from build123d import *

# Parameters (mm, degrees)
SKETCH1_W           = 60
SKETCH1_H           = 70
BOSS_EXTRUDE1_DEPTH = 5
SKETCH2_W           = 5
SKETCH2_H           = 70
BOSS_EXTRUDE2_DEPTH = 70
SKETCH3_R           = 2.5
CUT_EXTRUDE1_DEPTH  = 70
SKETCH4_R           = 11.5
CUT_EXTRUDE2_DEPTH  = 10
SKETCH5_R           = 1.5
CUT_EXTRUDE3_DEPTH  = 10


with BuildPart() as part:
    # Sketch1 → Boss-Extrude1 (new body)
    with BuildSketch(Plane(origin=(0, 0, 0), x_dir=(1, 0, 0), z_dir=(0, 1, 0))):
        Rectangle(SKETCH1_W, SKETCH1_H)
    extrude(amount=BOSS_EXTRUDE1_DEPTH)

    # Sketch2 → Boss-Extrude2 (add)
    with BuildSketch(Plane(origin=(0, 5, 0), x_dir=(1, 0, 0), z_dir=(0, 1, 0))):
        with Locations((27.5, 0)):
            Rectangle(SKETCH2_W, SKETCH2_H)
    extrude(amount=BOSS_EXTRUDE2_DEPTH)

    # Sketch3 → Cut-Extrude1 (cut)
    with BuildSketch(Plane(origin=(0, 5, 0), x_dir=(1, 0, 0), z_dir=(0, 1, 0))):
        with Locations(Location((0, 18.161512971, 0), (0, 0, 270))):
            Circle(SKETCH3_R)
        with Locations(Location((0, -18.161512971, 0), (0, 0, 90))):
            Circle(SKETCH3_R)
    extrude(amount=-CUT_EXTRUDE1_DEPTH, mode=Mode.SUBTRACT)

    # Sketch4 → Cut-Extrude2 (cut)
    with BuildSketch(Plane.ZY.offset(-25)):
        with Locations((0, 40)):
            Circle(SKETCH4_R)
    extrude(amount=-CUT_EXTRUDE2_DEPTH, mode=Mode.SUBTRACT)

    # Sketch5 → Cut-Extrude3 (cut)
    with BuildSketch(Plane.ZY.offset(-25)):
        with Locations((-15.5, 55.5)):
            Circle(SKETCH5_R)
        with Locations((15.5, 55.5)):
            Circle(SKETCH5_R)
        with Locations((15.5, 24.5)):
            Circle(SKETCH5_R)
        with Locations((-15.5, 24.5)):
            Circle(SKETCH5_R)
    extrude(amount=-CUT_EXTRUDE3_DEPTH, mode=Mode.SUBTRACT)


solid = part.part
Build history of the part. All positions in model axes, mm. A direction names the side the tool comes from. Coordinates: 2 decimals unless noted, no trailing zeros. Order: outer loops, then holes, each group sorted by start corner. A loop starts at its lowest first (then second) coordinate and runs counter-clockwise, first axis right, second up. Notation, with made-up numbers: M 78.5,1 L 97.5,1 A30 cw 97.5,40 Z; hole C 77,64.5 d6. An arc over 180 degrees is marked long. One line per question, with ' | ' between items. Start each with the question number.
Q1. Saw through at A-A (y = 55.5). List the corners of the cut face in (x, z).
Q2. Saw through at C-C (z = 0). List the corners of the cut face in (x, y), then the cut area to 3 significant figures.
Q3. 3-axis set-ups, long thin cutter, end or side, ignore diameter. For faces 1 (the face through (27.46, 55.57, -17)), 2 (the face through (25, 31.7, 8.3)): which of +Z, -Z, +X, -X, +Y, -Y reach the whole face in a straight line?
Q4. Probe L1, parallel to Y at x = 28.2, z = -15.5; L2, parallel to Y at x = 26.4, z = 0; L3, parallel to Y at x = 12.5, z = -4.5. List the from-to ranges inside material, lowest first. Write a range as from..to.
Q5. Saw through at B-B (y = 40). List the corners of the cut face in (x, z), then the cut area to 3 significant figures.
Q6. Saw through at D-D (z = -29). List the corners of the cut face in (x, y).
Q7. Two-plate mould, pull along X, no slides. Class faces 3 (the face through (-1.521, 2.535, -20.145)), 4 (the face through (1.521, 2.535, 20.145)), 5 (the face through (-30, 2, 0)), 6 (the face through (27, 21, 35)): +X half, -X half, draft (parallel to the pull), parting line (faces both ways), or undercut.
Q8. Flat gauge pins, fed straight in: pin 1 Ø3 at (x, z) = (23, 8) entering from -Y; pin 2 Ø20.5 at (y, z) = (40, 0) entering from +X; pin 3 Ø12 at (x, z) = (9.5, 1.5) entering from +Y; pin 4 Ø5 at (y, z) = (55.5, -15.5) entering from -X. Where does each tip first touch, or does it go through?
Check values:
1) outline: M 25,-35 L 30,-35 L 30,-17 L 25,-17 Z; M 25,-14 L 30,-14 L 30,14 L 25,14 Z; M 25,17 L 30,17 L 30,35 L 25,35 Z
2) outline: M -30,0 L 30,0 L 30,28.5 L 25,28.5 L 25,5 L -30,5 Z; M 25,51.5 L 30,51.5 L 30,75 L 25,75 Z | area: 535 mm2
3) face 1: +X, -X | face 2: +Z, -Z, -X, +Y
4) L1: y = 0..23, 26..54, 57..75 | L2: y = 0..28.5, 51.5..75 | L3: y = 0..5
5) outline: M 25,-35 L 30,-35 L 30,-11.5 L 25,-11.5 Z; M 25,11.5 L 30,11.5 L 30,35 L 25,35 Z | area: 235 mm2
6) outline: M -30,0 L 30,0 L 30,75 L 25,75 L 25,5 L -30,5 Z
7) face 3: undercut | face 4: undercut | face 5: -X half | face 6: draft
8) pin 1: stops at y = 0 | pin 2: passes through | pin 3: stops at y = 5 | pin 4: stops at x = 25
